from build123d import *

# Parameters (mm, degrees)
SKETCH_1_W               = 60
SKETCH_1_H               = 61
EXTRUDE_1_DEPTH          = 5
SKETCH_2_W               = 10
SKETCH_2_H               = 10
EXTRUDE_2_DEPTH          = 13
HOLE_WIZARD_2_D          = 3.3
SKETCH_9_R               = 2.85
EXTRUDE_3_DEPTH          = 3.5
SKETCH_5_W               = 1.75
SKETCH_5_H               = 18
HOLE_WIZARD_1_AT_2_COUNT = 2
HOLE_WIZARD_1_AT_2_PITCH = 51
HOLE_WIZARD_1_AT_3_COUNT = 2
HOLE_WIZARD_1_AT_3_PITCH = 71.421285343
HOLE_WIZARD_1_AT_4_COUNT = 2
HOLE_WIZARD_1_AT_4_PITCH = 50
HOLE_WIZARD_3_D          = 3.5


with BuildPart() as part:
    # 草图1 → 凸台-拉伸1 (new body)
    with BuildSketch(Plane(origin=(0, 0, 0), x_dir=(1, 0, 0), z_dir=(0, 1, 0))):
        with Locations((30, 30.5)):
            Rectangle(SKETCH_1_W, SKETCH_1_H)
    extrude(amount=EXTRUDE_1_DEPTH)

    # 草图2 → 凸台-拉伸2 (add)
    with BuildSketch(Plane.XZ):
        with Locations((5, -5)):
            Rectangle(SKETCH_2_W, SKETCH_2_H)
        with Locations((55, -5)):
            Rectangle(SKETCH_2_W, SKETCH_2_H)
        with Locations((55, -56)):
            Rectangle(SKETCH_2_W, SKETCH_2_H)
        with Locations((5, -56)):
            Rectangle(SKETCH_2_W, SKETCH_2_H)
    extrude(amount=EXTRUDE_2_DEPTH)

    # 孔2 (through all)
    with Locations(Plane(origin=(0, 5, 0), x_dir=(1, 0, 0), z_dir=(0, 1, 0))):
        with Locations((15, 58.5), (45, 58.5), (45, 2.5), (15, 2.5)):
            Hole(HOLE_WIZARD_2_D / 2)

    # 草图9 → 凸台-拉伸3 (add)
    with BuildSketch(Plane.XZ.offset(13)):
        with Locations(Location((5, -56, 0), (0, 0, 90))):
            Circle(SKETCH_9_R)
        with Locations(Location((55, -56, 0), (0, 0, 270))):
            Circle(SKETCH_9_R)
        with Locations(Location((55, -5, 0), (0, 0, 90))):
            Circle(SKETCH_9_R)
        with Locations(Location((5, -5, 0), (0, 0, 270))):
            Circle(SKETCH_9_R)
    extrude(amount=EXTRUDE_3_DEPTH)

    # 草图5 → 孔1 (revolve, cut)
    with BuildSketch(Plane(origin=(5, -13, -5), x_dir=(0, 0, -1), z_dir=(1, 0, 0))):
        with Locations((0.875, 9)):
            Rectangle(SKETCH_5_W, SKETCH_5_H)
    hole_wizard_1 = revolve(axis=Axis((5, 97, -5), (0, -1, 0)), mode=Mode.SUBTRACT)

    # 孔1 at 2: 孔1 ×2
    with Locations(*[(0, 0, -i * HOLE_WIZARD_1_AT_2_PITCH) for i in range(1, HOLE_WIZARD_1_AT_2_COUNT)]):
        add(hole_wizard_1, mode=Mode.SUBTRACT)

    # 孔1 at 3: 孔1 ×2
    with Locations(*[Vector(0.7000714109260575, 0, -0.7140728391445785) * (i * HOLE_WIZARD_1_AT_3_PITCH) for i in range(1, HOLE_WIZARD_1_AT_3_COUNT)]):
        add(hole_wizard_1, mode=Mode.SUBTRACT)

    # 孔1 at 4: 孔1 ×2
    with Locations(*[(i * HOLE_WIZARD_1_AT_4_PITCH, 0, 0) for i in range(1, HOLE_WIZARD_1_AT_4_COUNT)]):
        add(hole_wizard_1, mode=Mode.SUBTRACT)

    # 孔3 (through all)
    with Locations(Plane(origin=(0, -16.5, 0), x_dir=(-1, 0, 0), z_dir=(0, -1, 0))):
        with Locations((-5, 5), (-5, 56), (-55, 56), (-55, 5)):
            Hole(HOLE_WIZARD_3_D / 2)


solid = part.part
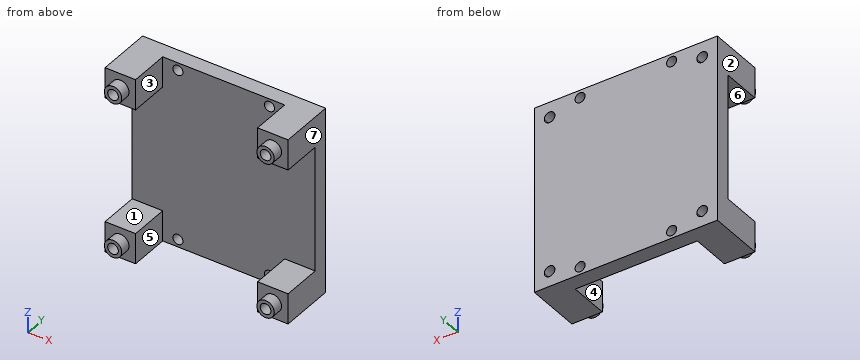
CAD build for the part. Positions are in the model's coordinates, mm. Face numbers are marked on the shaded views. A direction names the side the tool comes from. Coordinates: 2 decimals unless noted, no trailing zeros. Write each loop counter-clockwise with the first axis right and the second up, starting at its lowest first coordinate (ties: lowest second). Pieces come first, ordered by that corner, then holes. Notation, with made-up numbers: (64, 9.25) - (122, 9.25) arc R19 ccw to (122, 21.25) - close; hole circle Ø6 at (66.5, 89.5). An arc over 180 degrees is marked (long way). Use a Markdown table: item, result. Add a question column.
Item 1: Flat gauge pin, fed straight in: pin 1 (12 mm diameter, centred on x = 29, z = -13.5, fed in from -Y). Where does the tip first touch, or does it go through?
Item 2: Band-saw the part on A-A, the plane y = -10.25. Give the cut face in (x, z).
Item 3: Mould opens along X. For the marked faces 1, 2, 3 and 4 say: pulls with the +X half, pulls with the -X half, needs draft (parallel to the pull), parting line crosses it, or undercut.
Item 4: 3-axis set-ups, long thin cutter, end or side, ignore diameter. For the marked faces 5, 6 and 7: which of +Z, -Z, +X, -X, +Y, -Y reach the whole face in a straight line?
Item 5: Drill centre lines: L1, parallel to Z at x = 15, y = 3.25; L2, parallel to X at y = -14.5, z = -56; L3, parallel to Y at x = 44.5, z = -49. Where is each one in solid material? Low to high. Write a range as from..to.
Item 6: Band-saw the part on B-B, the plane x = 15. Give the cut face in (y, z), and give its area (3 significant figures).
Item 7: Band-saw the part on C-C, the plane y = -15. Give the cut face in (x, z).
Item 8: Band-saw the part on D-D, the plane z = -15.5. Give the cut face in (x, y), and give its area (3 significant figures).
Numbers:
| question | item | result |
|---|---|---|
| 1 | pin 1 | y = 0 |
| 2 | outline | (0, -61) - (10, -61) - (10, -51) - (0, -51) - close; (0, -10) - (10, -10) - (10, 0) - (0, 0) - close; (50, -61) - (60, -61) - (60, -51) - (50, -51) - close; (50, -10) - (60, -10) - (60, 0) - (50, 0) - close; hole circle Ø3.5 at (5, -56); hole circle Ø3.5 at (5, -5); hole circle Ø3.5 at (55, -56); hole circle Ø3.5 at (55, -5) |
| 3 | face 1 | needs draft |
| 3 | face 2 | pulls with the -X half |
| 3 | face 3 | undercut |
| 3 | face 4 | undercut |
| 4 | face 5 | +Z, -Z, -Y |
| 4 | face 6 | +X, -X, -Y |
| 4 | face 7 | +Z, -Z, +X, +Y, -Y |
| 5 | L1 | -61..-60.15, -56.85..-4.15, -0.85..0 |
| 5 | L2 | 2.15..3.25, 6.75..7.85, 52.15..53.25, 56.75..57.85 |
| 5 | L3 | 0..5 |
| 6 | outline | (0, -61) - (5, -61) - (5, -60.15) - (0, -60.15) - close; (0, -56.85) - (5, -56.85) - (5, -4.15) - (0, -4.15) - close; (0, -0.85) - (5, -0.85) - (5, 0) - (0, 0) - close |
| 6 | area | 272 mm2 |
| 7 | outline | circle Ø5.7 at (5, -56); circle Ø5.7 at (5, -5); circle Ø5.7 at (55, -56); circle Ø5.7 at (55, -5); hole circle Ø3.5 at (5, -56); hole circle Ø3.5 at (5, -5); hole circle Ø3.5 at (55, -56); hole circle Ø3.5 at (55, -5) |
| 8 | outline | (0, 0) - (60, 0) - (60, 5) - (0, 5) - close |
| 8 | area | 300 mm2 |
